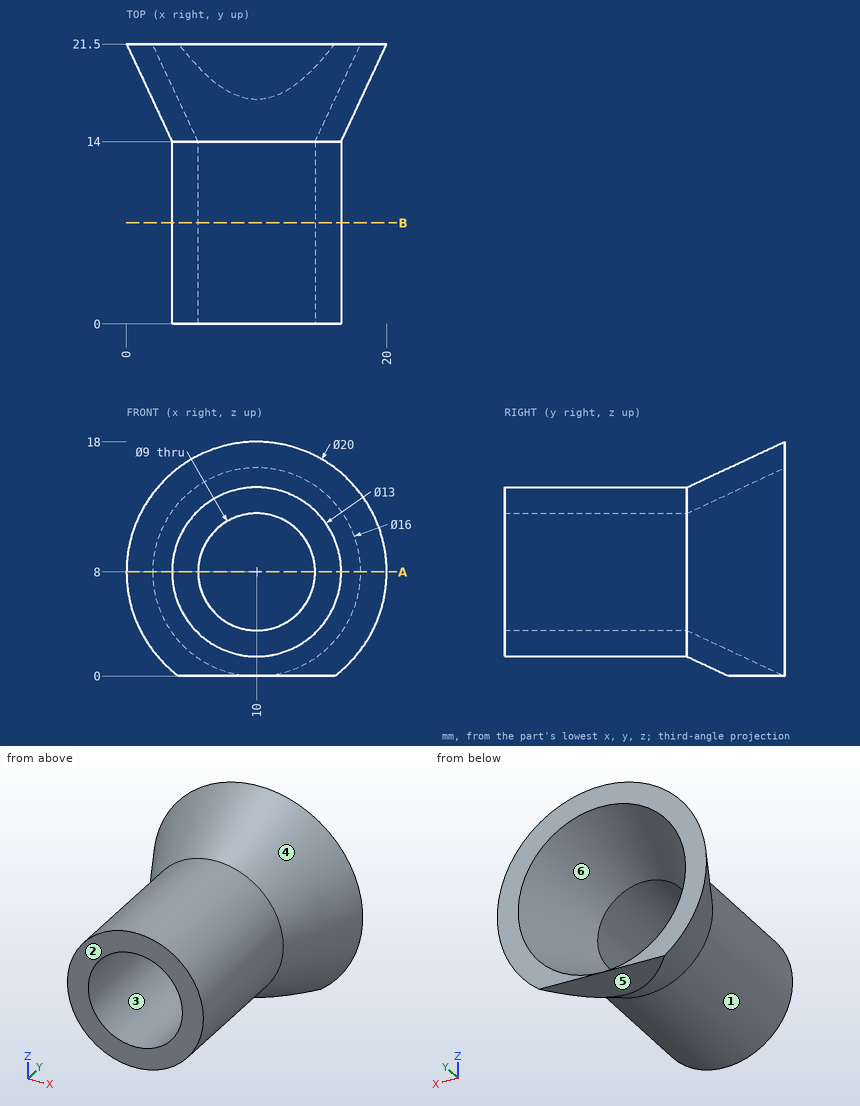
The drawing under review shows one solid part. Ordinate dimensions are in mm from its lowest x, y, z. A direction names the side the tool comes from. Round coordinates to 2 decimals unless told otherwise and drop trailing zeros. Loops run counter-clockwise (first coordinate to the right, second up) from the corner with the lowest first, then second, coordinate; pieces in that order, holes last. Notation, with made-up numbers: M 46.5,55 L 91.5,55 A13 cw 91.5,68 Z; hole C 12.5,78 d11. An arc over 180 degrees is marked long. Answer as CSV lines item,"result". Start each with the question number.
Item 1: Wall thickness on line 1 (X direction, y = 4.5, z = 8); line 2 (Z direction, x = 10, y = 6); line 3 (X direction, y = 19.75, z = 4.75): over which ranges is each line inside the solid? List them lowest first. Write a range as [from, to].
Item 2: Insertion check: P1, Ø10, axis at y = 16.5, z = 4, coming from the +X side; P2, Ø3, axis at x = 10.5, z = 12.5, coming from the -Y side; P3, Ø4, axis at y = 8, z = 3.5, coming from the +X side; P4, Ø8, axis at y = 15, z = 9, coming from the +X side. Each pin has a flat end and moves straight along its axis. Give the tip position at first contact, or say it passes through.
Item 3: Consider section B-B (y = 7.75). Write out the cut boundary in (x, z), then the cut area to 3 significant figures.
Item 4: For the marked faces 1 and 2, list the 3-axis set-ups (+Z, -Z, +X, -X, +Y, -Y) from which the entire face can be reached by the end or side of a thin tool; tool diameter is ignored.
Item 5: Mouldability with a two-part tool opening along X and no side actions: class the marked faces 3, 4, 5 and 6 as released by +X, released by -X, zero draft, split by the parting line, or undercut.
Item 6: Consider section A-A (z = 8). Write out the cut boundary in (x, y).
Answer:
1,line 1,"x = [3.5, 5.5], [14.5, 16.5]"
1,line 2,"z = [1.5, 3.5], [12.5, 14.5]"
1,line 3,"x = [1.41, 3.59], [16.41, 18.59]"
2,P1,"stops at x = 19.6"
2,P2,"stops at y = 0"
2,P3,"stops at x = 16"
2,P4,"stops at x = 18.8"
3,outline,"C 10,8 d13; hole C 10,8 d9"
3,area,"69.1 mm^2"
4,face 1,"-Y"
4,face 2,"+Z, -Z, +X, -X, -Y"
5,face 3,"undercut"
5,face 4,"split by the parting line"
5,face 5,"zero draft"
5,face 6,"undercut"
6,outline,"M 0,21.5 L 3.5,14 L 3.5,0 L 5.5,0 L 5.5,14 L 2,21.5 Z; M 14.5,0 L 16.5,0 L 16.5,14 L 20,21.5 L 18,21.5 L 14.5,14 Z"
